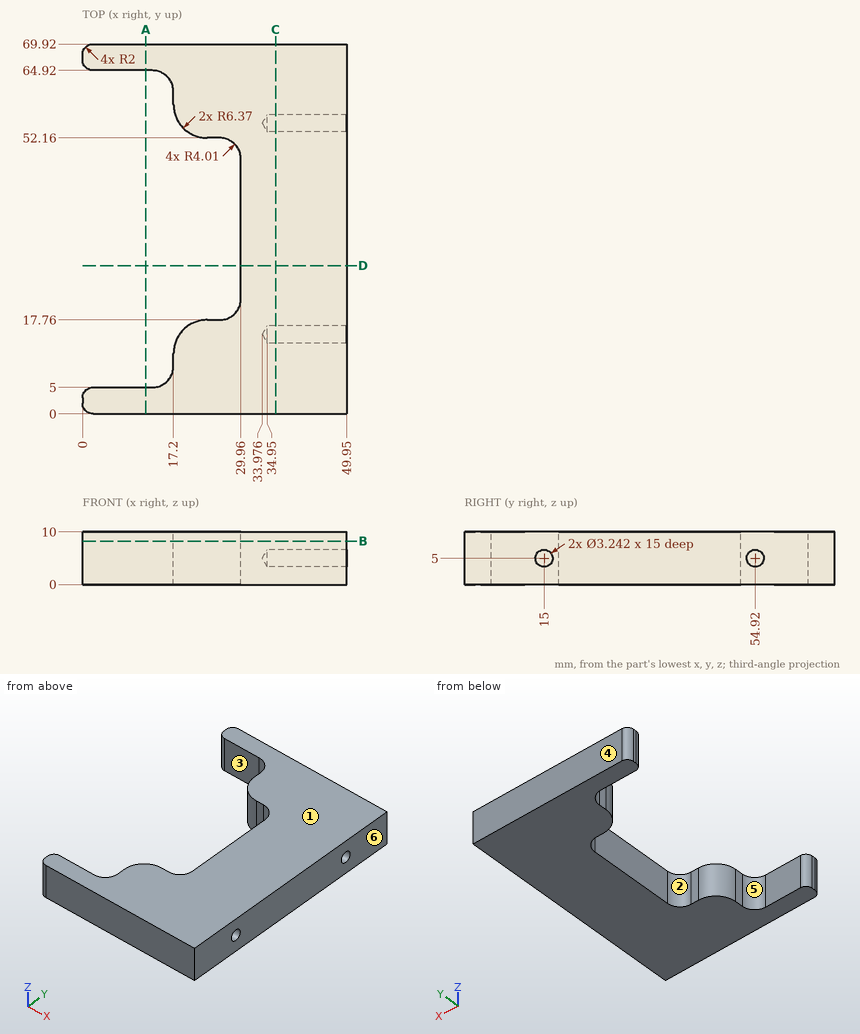
Geometry: see drawing. Coordinates: mm, zero at the bounding-box minimum. A direction names the side the tool comes from. Give positions to 0.01 mm unless a question says otherwise; leave off trailing zeros. Loops run counter-clockwise (first coordinate to the right, second up) from the corner with the lowest first, then second, coordinate; pieces in that order, holes last. Notation, with made-up numbers: (-24.5, 85) -> (-12.5, 85) arc R18 ccw to (-12.5, 109) -> close; hole circle Ø1 at (71, 27.5). An arc over 180 degrees is marked (long way). Answer as a JSON object with one key per item and string values. Group by question number.
Item 1: Line query: probe 1 along Y at (x, z) = (41.5, 5); probe 2 along Y at (x, z) = (25, 8.5); probe 3 along Y at (x, z) = (11, 0.5). Output: solid intervals per line, ascending.
Item 2: Cut plane D-D, the plane y = 28. Return the cut outline in (x, z), and give its area (3 significant figures).
Item 3: Pin query (flat end, axial travel): P1, Ø1.9, axis at y = 9.5, z = 3.5, coming from the -X side; P2, Ø4, axis at y = 27, z = 2.5, coming from the -X side; P3, Ø3, axis at y = 15, z = 5, coming from the +X side; P4, Ø8, axis at x = 27.5, y = 39, coming from the -Z side. Return the tip coordinate at first contact, or that it passes through.
Item 4: Cut plane A-A, the plane x = 12. Return the cut outline in (y, z), and give its area (3 significant figures).
Item 5: Pull-direction query (Y, two-part tool) for the marked faces 1, 2, 3 and 4; classes: released by +Y, released by -Y, zero draft, split by the parting line, or undercut.
Item 6: Cut plane C-C, the plane x = 36.5. Return the cut outline in (y, z), and give its area (3 significant figures).
Item 7: Reachability of the marked faces 5 and 6 from +Z, -Z, +X, -X, +Y, -Y: full face, straight path, thin tool, end or side. Return the list, or none.
Item 8: Cut plane B-B, the plane z = 8.25. Return the cut outline in (x, y), and give its area (3 significant figures).
Checks:
{
 "1": {"probe 1": "y = 0 to 13.38, 16.62 to 53.3, 56.54 to 69.92", "probe 2": "y = 0 to 17.76, 52.16 to 69.92", "probe 3": "y = 0 to 5, 64.92 to 69.92"},
 "2": {"outline": "(29.96, 0) -> (49.95, 0) -> (49.95, 10) -> (29.96, 10) -> close", "area": "200 mm²"},
 "3": {"P1": "stops at x = 17.17", "P2": "stops at x = 29.96", "P3": "stops at x = 34.88", "P4": "stops at z = 0"},
 "4": {"outline": "(0, 0) -> (5, 0) -> (5, 10) -> (0, 10) -> close; (64.92, 0) -> (69.92, 0) -> (69.92, 10) -> (64.92, 10) -> close", "area": "100 mm²"},
 "5": {"face 1": "zero draft", "face 2": "undercut", "face 3": "undercut", "face 4": "released by +Y"},
 "6": {"outline": "(0, 0) -> (69.92, 0) -> (69.92, 10) -> (0, 10) -> close; hole circle Ø3.24 at (15, 5); hole circle Ø3.24 at (54.92, 5)", "area": "683 mm²"},
 "7": {"face 5": "+Z, -Z, -X", "face 6": "+Z, -Z, +X, +Y, -Y"},
 "8": {"outline": "(0, 2) arc R2 ccw to (2, 0) -> (49.95, 0) -> (49.95, 69.92) -> (2, 69.92) arc R2 ccw to (0, 67.92) -> (0, 66.92) arc R2 ccw to (2, 64.92) -> (13.19, 64.92) arc R4.01 cw to (17.2, 60.91) -> (17.2, 58.53) arc R6.37 ccw to (23.57, 52.16) -> (25.95, 52.16) arc R4.01 cw to (29.96, 48.15) -> (29.96, 21.77) arc R4.01 cw to (25.95, 17.76) -> (23.57, 17.76) arc R6.37 ccw to (17.2, 11.39) -> (17.2, 9.01) arc R4.01 cw to (13.19, 5) -> (2, 5) arc R2 ccw to (0, 3) -> close", "area": "2,020 mm²"}
}
